from build123d import *

# Parameters (mm, degrees)
SKETCH1_R           = 5.9
BOSS_EXTRUDE1_DEPTH = 4
CUT_EXTRUDE2_DEPTH  = 3
CIRPATTERN1_COUNT   = 8


with BuildPart() as part:
    # Sketch1 → Boss-Extrude1 (new body)
    with BuildSketch(Plane.XY):
        Circle(SKETCH1_R)
    extrude(amount=BOSS_EXTRUDE1_DEPTH)

    # Sketch2 → Cut-Extrude2 (cut)
    with BuildSketch(Plane(origin=(0, 0, 0), x_dir=(-1, 0, 0), z_dir=(0, 0, -1))):
        with BuildLine():
            Line((1, 5.814636704), (1, 2.93428015))
            Line((1, 2.93428015), (-1, 2.93428015))
            Line((-1, 2.93428015), (-1, 5.814636704))
            ThreePointArc((-1, 5.814636704), (0, 5.9), (1, 5.814636704))
        make_face()
    cut_extrude2 = extrude(amount=-CUT_EXTRUDE2_DEPTH, mode=Mode.SUBTRACT)

    # CirPattern1: Cut-Extrude2 ×8 about axis
    cirpattern1_axis = Axis((0, 0, 0), (0, 0, 1))
    for i in range(1, CIRPATTERN1_COUNT):
        add(cut_extrude2.rotate(cirpattern1_axis, i * 360 / CIRPATTERN1_COUNT), mode=Mode.SUBTRACT)


solid = part.part
Source: CAD feature listing. Evaluate the final solid. Frame: model axes, mm. A direction names the side the tool comes from. Give positions to 0.01 mm unless a question says otherwise; leave off trailing zeros. Loops run counter-clockwise (first coordinate to the right, second up) from the corner with the lowest first, then second, coordinate; pieces in that order, holes last. Notation, with made-up numbers: (-16.75, -5.5) -> (25.25, -5.5) arc R17 ccw to (25.25, 5.5) -> close; hole circle Ø10 at (20, 34). An arc over 180 degrees is marked (long way). Use a Markdown table: item, result. Add a question column.
1) First-contact query: pin 1 (1 mm diameter, centred on x = 0.5, y = 3, fed in from -Z); pin 2 (1 mm diameter, centred on y = 0, z = 1, fed in from -X); pin 3 (0.6 mm diameter, centred on x = 0, y = 4.5, fed in from -Z); pin 4 (1 mm diameter, centred on x = 0, z = 1.5, fed in from -Y). Flat tips, straight axial feed; report the tip coordinate or a pass-through.
2) Line query: line 1 along Y through (x, z) = (-3, 1.35); line 2 along Y through (x, z) = (-1.5, 1.2); line 3 along Y through (x, z) = (-1.75, 2.15). Output: solid intervals per line, ascending. Write a range as [from, to].
3) Section query A-A, the plane x = 0. Return the cut outline in (y, z), then the cut area to 3 significant figures.
4) Reachability of faces 1 (the face through (4, 0, 3)), 2 (the face through (-2.085, 2.065, 1.479)), 3 (the face through (-1, 4, 1)), 4 (the face through (-2.934, 0, 1)) from +Z, -Z, +X, -X, +Y, -Y: full face, straight path, thin tool, end or side. Return the list, or none.
5) Pull-direction query (Y, two-part tool) for faces 5 (the face through (2.934, 0, 1)), 6 (the face through (0, 0, 4)), 7 (the face through (0, 2.934, 1)); classes: +Y half, -Y half, draft (parallel to the pull), parting line (faces both ways), or undercut.
6) Section query D-D, the plane x = -2.5. Return the cut outline in (y, z).
Numbers:
| question | item | result |
|---|---|---|
| 1 | pin 1 | stops at z = 0 |
| 1 | pin 2 | stops at x = -2.93 |
| 1 | pin 3 | stops at z = 3 |
| 1 | pin 4 | stops at y = -2.93 |
| 2 | line 1 | y = [-5.08, -4.41], [-1.59, -1], [1, 1.59], [4.41, 5.08] |
| 2 | line 2 | y = [-5.71, -2.91], [-2.65, 2.65], [2.91, 5.71] |
| 2 | line 3 | y = [-5.63, -3.16], [-2.4, 2.4], [3.16, 5.63] |
| 3 | outline | (-5.9, 3) -> (-2.93, 3) -> (-2.93, 0) -> (2.93, 0) -> (2.93, 3) -> (5.9, 3) -> (5.9, 4) -> (-5.9, 4) -> close |
| 3 | area | 29.4 mm2 |
| 4 | face 1 | -Z, +X |
| 4 | face 2 | -Z |
| 4 | face 3 | -Z, +Y |
| 4 | face 4 | -Z, -X |
| 5 | face 5 | undercut |
| 5 | face 6 | draft |
| 5 | face 7 | +Y half |
| 6 | outline | (-5.34, 0) -> (-3.91, 0) -> (-3.91, 3) -> (-1.65, 3) -> (-1.65, 0) -> (1.65, 0) -> (1.65, 3) -> (3.91, 3) -> (3.91, 0) -> (5.34, 0) -> (5.34, 4) -> (-5.34, 4) -> close |
